Design review of the part built by this model. Coordinates are the model's own, in mm. Coordinates: 2 decimals unless noted, no trailing zeros. Write each loop counter-clockwise with the first axis right and the second up, starting at its lowest first coordinate (ties: lowest second). Pieces come first, ordered by that corner, then holes.
Q1. For L1, parallel to Y at x = 41, z = 2.1; L2, parallel to Y at x = 20, z = 1.25; L3, parallel to Y at x = 69, z = 2.8, list the stretches that pass through material, from the lowest coordinate up.
Q2. Take a section at B-B, the plane x = 45. Write out the cut boundary in (y, z), plus the area to 3 significant figures.
Q3. Take a section at A-A, the plane x = 18. Write out the cut boundary in (y, z).
Q4. For pin 1 Ø0.9 at (x, z) = (63, 2) entering from +Y; pin 2 Ø0.9 at (y, z) = (40, 2) entering from +X; pin 3 Ø1.5 at (x, z) = (79.5, 2) entering from -Y, all flat-tipped, find the tip position at first contact; note any pin that passes through.
Q5. Take a section at C-C, the plane y = 75. Write out the cut boundary in (x, z).
Q6. Take a section at D-D, the plane z = 1.35. State how many separate pieces and enclosed holes the cut face has, plus the area to 3 significant figures.
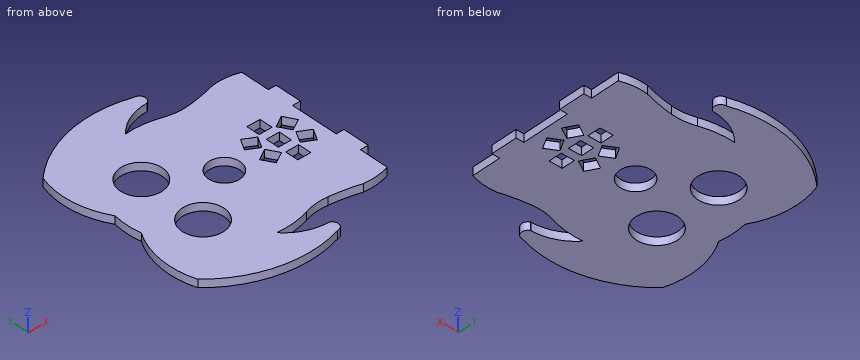
from build123d import *

# Parameters (mm, degrees)
SKETCH2_R           = 8
SKETCH2_R_2         = 6
SKETCH2_W           = 5
SKETCH2_H           = 5
BOSS_EXTRUDE1_DEPTH = 3


with BuildPart() as part:
    # Sketch2 → Boss-Extrude1 (new body)
    with BuildSketch(Plane.XY):
        with BuildLine():
            Line((81.032103119, 50.181312), (81.032103119, 60.181312))
            Line((81.032103119, 60.181312), (78.032103119, 60.181312))
            Line((78.032103119, 60.181312), (78.032103119, 71.181312))
            ThreePointArc((78.032103119, 71.181312), (73.050090858, 72.33654353), (67.936161846, 72.284235691))
            ThreePointArc((67.936161846, 72.284235691), (62.235942644, 70.892785416), (56.438402104, 69.988818319))
            ThreePointArc((56.438402104, 69.988818319), (51.886102873, 69.971964975), (47.437133801, 70.93653043))
            ThreePointArc((47.437133801, 70.93653043), (41.102316828, 72.343050119), (34.613643935, 72.416041905))
            ThreePointArc((34.613643935, 72.416041905), (40.990344282, 77.154811793), (48.755286163, 78.83526559))
            ThreePointArc((48.755286163, 78.83526559), (48.80614848, 78.851120911), (48.85704212, 78.866875402))
            ThreePointArc((48.85704212, 78.866875402), (50.134187725, 81.487874692), (47.847872498, 83.297156554))
            ThreePointArc((47.847872498, 83.297156554), (24.351235249, 84.294658733), (3.641458375, 73.150507154))
            ThreePointArc((3.641458375, 73.150507154), (2.19654611, 59.548103084), (6.61028157, 46.600821237))
            ThreePointArc((6.61028157, 46.600821237), (6.138572184, 41.181312), (6.61028157, 35.761802763))
            ThreePointArc((6.61028157, 35.761802763), (2.19654611, 22.814520916), (3.641458375, 9.212116846))
            ThreePointArc((3.641458375, 9.212116846), (24.351235249, -1.932034733), (47.847872498, -0.934532554))
            ThreePointArc((47.847872498, -0.934532554), (50.134187725, 0.874749308), (48.85704212, 3.495748598))
            ThreePointArc((48.85704212, 3.495748598), (48.80614848, 3.511503089), (48.755286163, 3.52735841))
            ThreePointArc((48.755286163, 3.52735841), (40.990344282, 5.207812207), (34.613643935, 9.946582095))
            ThreePointArc((34.613643935, 9.946582095), (41.102316828, 10.019573881), (47.437133801, 11.42609357))
            ThreePointArc((47.437133801, 11.42609357), (51.886102873, 12.390659025), (56.438402104, 12.373805681))
            ThreePointArc((56.438402104, 12.373805681), (62.235942644, 11.469838584), (67.936161846, 10.078388309))
            ThreePointArc((67.936161846, 10.078388309), (73.050090858, 10.02608047), (78.032103119, 11.181312))
            Line((78.032103119, 11.181312), (78.032103119, 22.181312))
            Line((78.032103119, 22.181312), (81.032103119, 22.181312))
            Line((81.032103119, 22.181312), (81.032103119, 32.181312))
            Line((81.032103119, 32.181312), (78.032103119, 32.181312))
            Line((78.032103119, 32.181312), (78.032103119, 50.181312))
            Line((78.032103119, 50.181312), (81.032103119, 50.181312))
        make_face()
        with Locations((23.507028058, 53.931312)):
            Circle(SKETCH2_R, mode=Mode.SUBTRACT)
        with Locations((43.507028058, 41.181312)):
            Circle(SKETCH2_R_2, mode=Mode.SUBTRACT)
        with Locations((23.507028058, 28.431312)):
            Circle(SKETCH2_R, mode=Mode.SUBTRACT)
        with Locations((64.423022125, 41.181312)):
            Rectangle(SKETCH2_W, SKETCH2_H, mode=Mode.SUBTRACT)
        with Locations((64.423022125, 33.181312)):
            Rectangle(SKETCH2_W, SKETCH2_H, mode=Mode.SUBTRACT)
        Polygon((72.266288865, 48.59637551), (67.936161846, 46.09637551), (70.436161846, 41.766248491), (74.766288865, 44.266248491), align=None, mode=Mode.SUBTRACT)
        Polygon((67.936161846, 36.266248491), (72.266288865, 33.766248491), (74.766288865, 38.09637551), (70.436161846, 40.596375509), align=None, mode=Mode.SUBTRACT)
        with Locations((64.423022125, 49.181312)):
            Rectangle(SKETCH2_W, SKETCH2_H, mode=Mode.SUBTRACT)
        Polygon((56.579755385, 33.766248491), (60.909882404, 36.266248491), (58.409882404, 40.59637551), (54.079755385, 38.09637551), align=None, mode=Mode.SUBTRACT)
        Polygon((60.909882404, 46.09637551), (56.579755385, 48.596375509), (54.079755385, 44.266248491), (58.409882404, 41.766248491), align=None, mode=Mode.SUBTRACT)
    extrude(amount=BOSS_EXTRUDE1_DEPTH)


solid = part.part
Responses:
1. L1: y = -2.55 to 5.2, 10.01 to 35.73, 46.63 to 72.35, 77.16 to 84.91
1. L2: y = -0.7 to 21.24, 35.62 to 46.74, 61.12 to 83.06
1. L3: y = 9.97 to 35.65, 38.11 to 44.25, 46.71 to 72.4
2. outline: (-1.74, 0) - (3.91, 0) - (3.91, 3) - (-1.74, 3) - close; (10.72, 0) - (35.37, 0) - (35.37, 3) - (10.72, 3) - close; (46.99, 0) - (71.64, 0) - (71.64, 3) - (46.99, 3) - close; (78.46, 0) - (84.11, 0) - (84.11, 3) - (78.46, 3) - close
2. area: 182 mm2
3. outline: (0.04, 0) - (22.63, 0) - (22.63, 3) - (0.04, 3) - close; (34.23, 0) - (48.13, 0) - (48.13, 3) - (34.23, 3) - close; (59.73, 0) - (82.33, 0) - (82.33, 3) - (59.73, 3) - close
4. pin 1: stops at y = 71.15
4. pin 2: stops at x = 78.03
4. pin 3: stops at y = 22.18
5. outline: (5.71, 0) - (37.38, 0) - (37.38, 3) - (5.71, 3) - close
6. separate pieces: 1
6. enclosed holes: 10
6. area: 4,730 mm2
